Design review of the part built by this model. Coordinates are the model's own, in mm. Face numbers are marked on the shaded views. Coordinates: 2 decimals unless noted, no trailing zeros. Use one line per item in the form item = value. Start each with the question number.
(1) For L1, parallel to Z at x = -46, y = 0.3; L2, parallel to X at y = 4.4, z = -41; L3, parallel to Y at x = -107.5, z = 11, list the stretches that pass through material, from the lowest coordinate up.
(2) The part is to be moulded in two halves that separate along Z. For the marked faces 1 and 2, say which applies: pulls with the +Z half, pulls with the -Z half, needs draft (parallel to the pull), parting line crosses it, or undercut.
(3) Clearance check with flat-ended pins moving along their axes: pin 1 Ø5.5 at (x, z) = (27.85, -15) entering from -Y; pin 2 Ø5 at (x, z) = (-302.61, -14.48) entering from +Y. State where each tip first meets the part, or that it passes through.
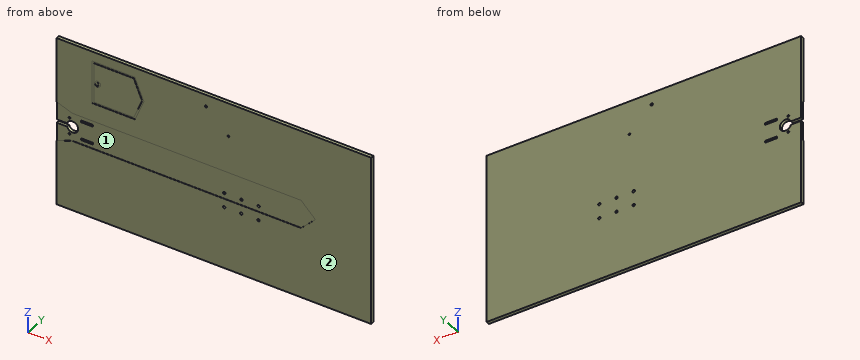
Autodesk Inventor part; units mm, degrees
ref_plane "YZ Plane" through (0, 0, 0) normal (1, 0, 0) x (0, 1, 0)
ref_plane "XZ Plane" through (0, 0, 0) normal (0, 1, 0) x (-1, 0, 0)
ref_plane "XY Plane" through (0, 0, 0) normal (0, 0, 1) x (1, 0, 0)
sketch "Эскиз1" plane through (0, 0, 0) normal (0, 1, 0) x (-1, 0, 0)
  ellipse E0 centre (50, 0) end of major axis (50, -150) minor radius 275
  line L0 (50, 150) -> (-225, 150)
  line L1 (-225, 150) -> (-225, -150)
  line L2 (-225, -150) -> (50, -150)
  line L3 (50, -150) -> (50, 150)
  line L4 (50, 150) -> (325, 150)
  line L5 (325, 150) -> (325, -150)
  line L6 (325, -150) -> (50, -150)
  line L7 (50, -150) -> (50, 150)
  point P0 (0, 0)
  point P1 (50, -150)
  point P2 (50, 0)
  dimension "d0" = 275
  dimension "d1" = 150
  dimension "d40" = 325
extrude "Выдавливание1" add sketch "Эскиз1" along normal blind 6
sketch "Эскиз2" plane through (0, 0, 0) normal (0, -1, 0) x (1, 0, 0)
  line L0 (-260, 60) -> (-190, 60)
  line L1 (-190, 60) -> (-190, 130)
  line L2 (-190, 130) -> (-260, 130)
  line L3 (-260, 130) -> (-260, 60)
  line L4 (-190, 60) -> (-175.5025, 95)
  line L5 (-175.5025, 95) -> (-190, 130)
  line L6 (-325, 150) -> (225, 150)
  line L7 (-325, 150) -> (225, 150)
  line L8 (-250, 190) -> (-331.0569, 190) construction
  line L9 (-175.5025, 51.7755) -> (-260, 130) construction
  line L10 (-260, 60) -> (-175.5025, 138.2245) construction
  circle A0 centre (-222.1933, 95) radius 14.4069 construction
  line L11 (-187.9955, 133) -> (-263, 133)
  line L12 (-263, 133) -> (-263, 57)
  line L13 (-263, 57) -> (-187.9955, 57)
  line L14 (-187.9955, 133) -> (-172.2553, 95)
  line L15 (-172.2553, 95) -> (-187.9955, 57)
  line L16 (-260, 95) -> (-253, 95)
  circle A1 centre (-253, 95) radius 5
  circle A2 centre (-253, 96.75) radius 0.75
  circle A3 centre (-253, 93.25) radius 0.75
  line L17 (-253, 93.25) -> (-253, 96.75)
  line L18 (-325, -150) -> (-325, 150)
  line L19 (-325, -150) -> (-325, 150)
  line L20 (-325, 35) -> (-297.5252, 25)
  line L21 (-297.5252, 25) -> (102.4748, 25)
  line L22 (102.4748, 25) -> (127.4748, 0)
  line L23 (225, 150) -> (225, -150)
  line L24 (225, 0) -> (-325, 0) construction
  line L25 (-325, -35) -> (-297.5252, -25)
  line L26 (-297.5252, -25) -> (102.4748, -25)
  line L27 (102.4748, -25) -> (127.4748, 0)
  point P0 (-325, -115)
  point P1 (-325, 115)
  point P2 (-331.0569, 190)
  dimension "d12" = 135
  dimension "d13" = 70
  dimension "d16" = 3
  dimension "d17" = 3
  dimension "d20" = 7
  dimension "d21" = 10
  dimension "d35" = 55
  dimension "d37" = 1.75
  dimension "d38" = 1.5
  dimension "d57" = 62
  dimension "d59" = 70
  dimension "d60" = 135
  dimension "d62" = 400
  dimension "d63" = 35
  dimension "d64" = 25
  dimension "d65" = 32
extrude "Выдавливание2" cut sketch "Эскиз2" against normal blind 0.5
sketch "Эскиз3" plane through (0, 0, 0) normal (0, -1, 0) x (1, 0, 0)
  circle A0 centre (-297.5252, 0) radius 10
  line L0 (-295, -14.0809) -> (-297.5252, 0) construction
  circle A1 centre (-302.6052, -14.48) radius 1.6
  line L1 (-325, -35) -> (-325, 35)
  line L2 (-325, 0) -> (327.0887, 0) construction
  line L3 (-305.9052, -17.78) -> (-261.4552, -17.78)
  line L4 (-261.4552, -17.78) -> (-261.4552, 17.78)
  line L5 (-261.4552, 17.78) -> (-305.9052, 17.78)
  line L6 (-305.9052, 17.78) -> (-305.9052, -17.78)
  line L7 (-261.4552, -17.78) -> (-285.6608, 0) construction
  line L8 (-261.4552, 17.78) -> (-285.6608, 0) construction
  line L9 (-261.4552, 17.78) -> (-282.4372, 17.78)
  line L10 (-282.4372, 17.78) -> (-282.4372, 14.418)
  line L11 (-282.4372, 14.418) -> (-261.4552, 14.418)
  line L12 (-261.4552, 14.418) -> (-261.4552, 17.78)
  line L13 (-282.4372, -17.78) -> (-282.4372, -14.418)
  line L14 (-282.4372, -14.418) -> (-261.4552, -14.418)
  circle A2 centre (-302.6052, 14.48) radius 1.6
  line L15 (-297.5252, -25) -> (-325, -35)
  line L16 (102.4748, -25) -> (-297.5252, -25)
  line L17 (-325, 35) -> (-297.5252, 25)
  line L18 (-297.5252, 25) -> (102.4748, 25)
  line L19 (-297.5252, 25) -> (102.4748, 25)
  line L20 (-297.5252, -25) -> (-297.5252, 25) construction
  line L21 (-307.0646, 3) -> (-325, 3)
  line L22 (-307.0646, -3) -> (-325, -3)
  point P0 (0, 0)
  point P1 (-325, 25)
  point P2 (-305.9052, 5.4567)
  point P3 (-305.9052, -5.4567)
  point P4 (-282.4372, 17.78)
  dimension "d22" = 20
  dimension "d23" = 5.08
  dimension "d25" = 14.48
  dimension "d26" = 3.2
  dimension "d28" = 44.45
  dimension "d29" = 35.56
  dimension "d30" = 8.38
  dimension "d31" = 3.362
  dimension "d32" = 20.982
  dimension "d67" = 3
extrude "Выдавливание3" cut sketch "Эскиз3" against normal blind 14.48 contours A0 L6 | A0 L22 L1 L21 | A0 L6 | L5 L4 L11 L10 | L13 L14 L4 L3 | A1 | A2
sketch "Эскиз4" plane through (0, 0, 0) normal (0, -1, 0) x (1, 0, 0)
  line L0 (0, 0) -> (-4.3, 0) construction
  line L1 (-4.3, 0) -> (-4.3, -50) construction
  line L2 (-4.3, -50) -> (0, -50) construction
  line L3 (0, -50) -> (0, 0) construction
  circle A0 centre (-2.15, -15) radius 2.15
  circle A1 centre (-2.15, -40) radius 2.15
  line L4 (-30, 0) -> (-34.3, 0) construction
  line L5 (-34.3, 0) -> (-34.3, -50) construction
  line L6 (-34.3, -50) -> (-30, -50) construction
  line L7 (-30, -50) -> (-30, 0) construction
  circle A2 centre (-32.15, -15) radius 2.15
  circle A3 centre (-32.15, -40) radius 2.15
  line L8 (30, 0) -> (25.7, 0) construction
  line L9 (25.7, 0) -> (25.7, -50) construction
  line L10 (25.7, -50) -> (30, -50) construction
  line L11 (30, -50) -> (30, 0) construction
  circle A4 centre (27.85, -15) radius 2.15
  circle A5 centre (27.85, -40) radius 2.15
  line L12 (0, 0) -> (-4.3, 0) construction
  line L13 (-4.3, 0) -> (-4.3, -50) construction
  line L14 (-4.3, -50) -> (0, -50) construction
  line L15 (0, -50) -> (0, 0) construction
  circle A6 centre (-2.15, -15) radius 2.15
  circle A7 centre (-2.15, -40) radius 2.15
  circle A8 centre (-63.7357, 129.0861) radius 2.1
  circle A9 centre (-24.6255, 90.6066) radius 1.6
  dimension "d41" = 4.3
  dimension "d42" = 50
  dimension "d43" = 10
  dimension "d44" = 15
  dimension "d47" = 30
  dimension "d50" = 30
  dimension "d53" = 4.2
  dimension "d54" = 3.2
extrude "Выдавливание4" cut sketch "Эскиз4" against normal blind 10
equation "\"d33\" = d25"
properties part number "щиток"
Computed values:
q1.L1 = -150 to -25, 25 to 150
q1.L2 = -325 to -34.05, -30.25 to -4.05, -0.25 to 25.95, 29.75 to 225
q1.L3 = 0.5 to 6
q2.face_1 = undercut
q2.face_2 = needs draft
q3.pin_1 = 0.5
q3.pin_2 = 6
